Verification items for this drawing (mm, ordinates from the low corner). A direction names the side the tool comes from. Coordinates: 2 decimals unless noted, no trailing zeros. Loops run counter-clockwise (first coordinate to the right, second up) from the corner with the lowest first, then second, coordinate; pieces in that order, holes last.
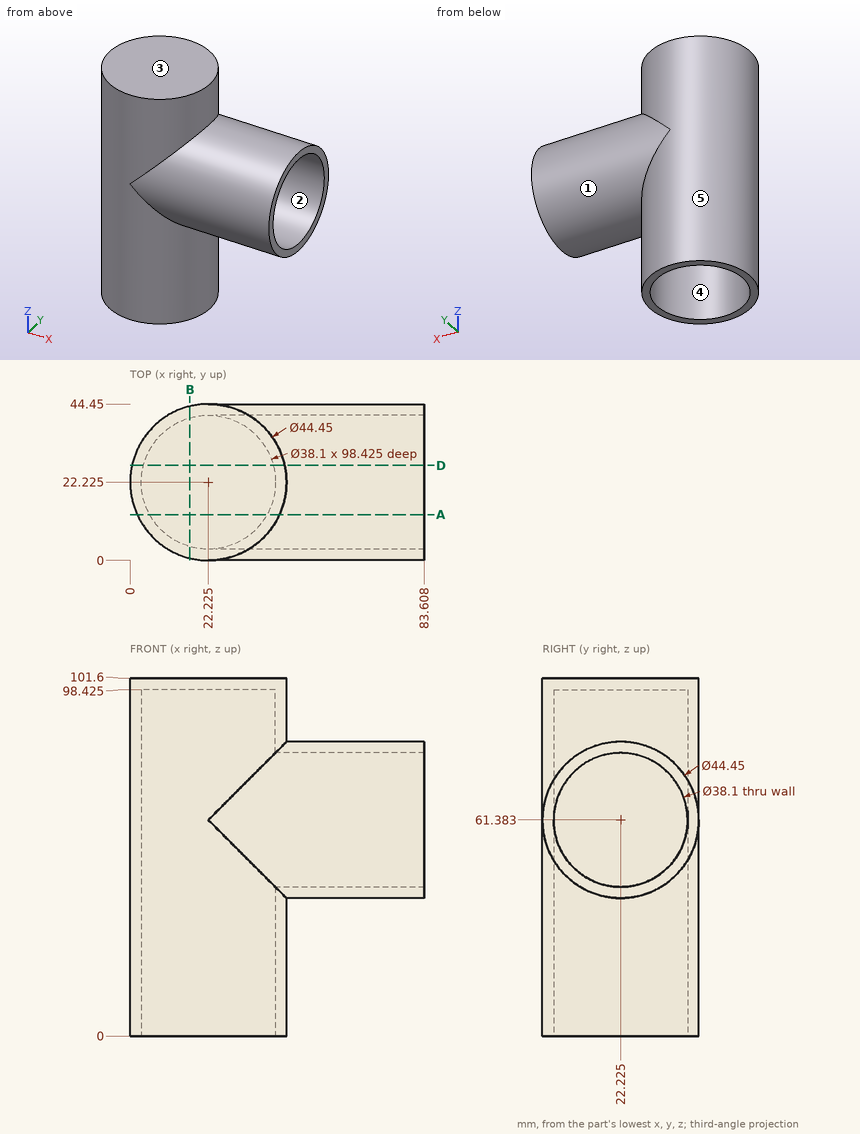
(1) Section check D-D, the plane y = 27. Enter the section's corners in (x, z) (1 decimal), plus the area to 3 significant figures.
(2) Draft check along Y on the marked faces 1, 2 and 3. Enter one of: pulls with the +Y half, pulls with the -Y half, needs draft (parallel to the pull), parting line crosses it, or undercut.
(3) Gauge pin test, flat ends, axial feed: P1, Ø3, axis at x = 10.5, z = 24, coming from the -Y side; P2, Ø1, axis at x = 64, z = 43.5, coming from the +Y side; P3, Ø1, axis at y = 35, z = 75.5, coming from the -X side; P4, Ø4, axis at x = 71, z = 87, coming from the +Y side. Record the tip position at first contact, or that the pin passes through.
(4) Scan lines: line 1 along Z through (x, y) = (71, 22.5) (1 decimal); line 2 along Z through (x, y) = (8.5, 13) (1 decimal); line 3 along Y through (x, z) = (74.5, 74.5) (1 decimal). Record each from-to range of solid material in increasing order.
(5) Section check A-A, the plane y = 13. Enter the section's corners in (x, z) (1 decimal), plus the area to 3 significant figures.
(6) Section check B-B, the plane x = 17. Enter the section's corners in (y, z) (1 decimal).
(7) Set-up check for the marked faces 4 and 5: record each of +Z, -Z, +X, -X, +Y, -Y from which the full face is reachable in a straight line by a thin tool's end or side.
Determined:
1. outline: (0.5, 0) - (3.8, 0) - (3.8, 98.4) - (40.7, 98.4) - (40.7, 79.8) - (83.6, 79.8) - (83.6, 83.1) - (43.9, 83.1) - (43.9, 101.6) - (0.5, 101.6) - close; (40.7, 0) - (43.9, 0) - (43.9, 39.7) - (83.6, 39.7) - (83.6, 42.9) - (40.7, 42.9) - close
1. area: 919 mm2
2. face 1: parting line crosses it
2. face 2: undercut
2. face 3: needs draft
3. P1: stops at y = 2.49
3. P2: stops at y = 36.07
3. P3: stops at x = 3.7
3. P4: passes through
4. line 1: z = 39.2 to 42.3, 80.4 to 83.6
4. line 2: z = 98.4 to 101.6
4. line 3: y = 4.3 to 8.4, 36 to 40.2
5. outline: (2, 0) - (5.6, 0) - (5.6, 98.4) - (38.9, 98.4) - (38.9, 78.1) - (83.6, 78.1) - (83.6, 81.6) - (42.4, 81.6) - (42.4, 101.6) - (2, 101.6) - close; (38.9, 0) - (42.4, 0) - (42.4, 41.2) - (83.6, 41.2) - (83.6, 44.7) - (38.9, 44.7) - close
5. area: 1,000 mm2
6. outline: (0.6, 0) - (3.9, 0) - (3.9, 98.4) - (40.5, 98.4) - (40.5, 0) - (43.8, 0) - (43.8, 101.6) - (0.6, 101.6) - close
7. face 4: -Z
7. face 5: none
